Input: dimensioned drawing with shaded views. Units: mm. Origin: part minimum x, y, z. A direction names the side the tool comes from. Give positions to 0.01 mm unless a question says otherwise; leave off trailing zeros. Write each loop counter-clockwise with the first axis right and the second up, starting at its lowest first coordinate (ties: lowest second). Pieces come first, ordered by that corner, then holes. Notation, with made-up numbers: (24, 20.5) -> (46, 20.5) arc R19 cw to (46, 33.5) -> close; hole circle Ø8 at (24, 28.5). An arc over 180 degrees is marked (long way). Answer as a JSON object with one key per item and string values.
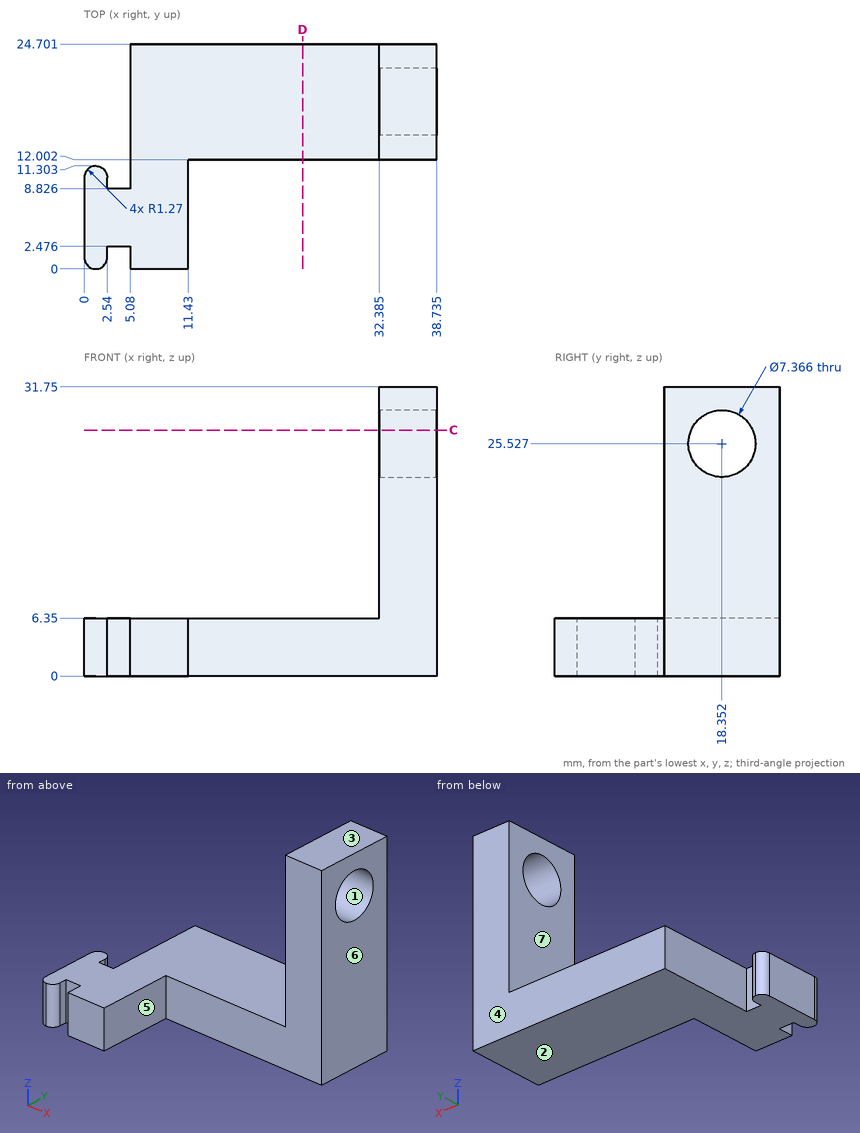
Q1. Material intervals for L1, parallel to X at y = 22.5, z = 21 (1 decimal); L2, parallel to Z at x = 22.5, y = 16.75; L3, parallel to Y at x = 35.5, z = 17.5, sorted ascending. Write a range as from..to.
Values:
{"L1": "32.4..38.7", "L2": "0..6.35", "L3": "12..24.7"}
Q2. Cut plane D-D (x = 24). Return the cut outline in (y, z).
Values:
{"outline": "(12, 0) -> (24.7, 0) -> (24.7, 6.35) -> (12, 6.35) -> close"}
Q3. Set-up query: the marked faces 5, 6 and 7. Return all of +Z, -Z, +X, -X, +Y, -Y with unobstructed straight access to the full face (end or side cutting, diameter ignored); none if empty.
Values:
{"face 5": "+Z, -Z, +X, -Y", "face 6": "+Z, -Z, +X, +Y, -Y", "face 7": "+Z, -X, +Y, -Y"}
Q4. First-contact query: P1, Ø3, axis at x = 6.5, y = 9.5, coming from the +Z side; P2, Ø4.5, axis at y = 18.35, z = 25.53, coming from the +X side; P3, Ø6.5, axis at y = 16.5, z = 23.5, coming from the -X side (1 decimal); P4, Ø3, axis at y = 18, z = 1.5, coming from the -X side. Flat tips, straight axial feed; report the tip coordinate or a pass-through.
Values:
{"P1": "z = 6.35", "P2": "through", "P3": "x = 32.4", "P4": "x = 5.08"}
Q5. Mould query, pull axis Z, two halves, no side actions, for the marked faces 1, 2, 3 and 4. Classes: pulls with the +Z half, pulls with the -Z half, needs draft (parallel to the pull), parting line crosses it, or undercut.
Values:
{"face 1": "undercut", "face 2": "pulls with the -Z half", "face 3": "pulls with the +Z half", "face 4": "needs draft"}
Q6. Cut plane C-C (z = 27). Return the cut outline in (x, y) (1 decimal).
Values:
{"outline": "(32.4, 12) -> (38.7, 12) -> (38.7, 15) -> (32.4, 15) -> close; (32.4, 21.7) -> (38.7, 21.7) -> (38.7, 24.7) -> (32.4, 24.7) -> close"}
